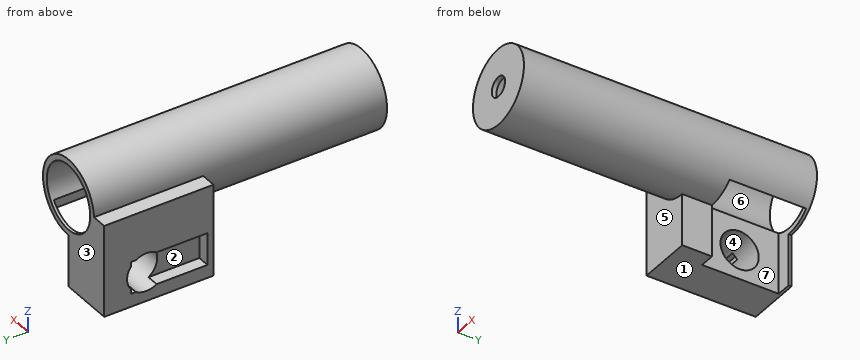
```python
from build123d import *

# Parameters (mm, degrees)
F0_R      = 25
F1_DEPTH  = 200
F4_W      = 35
F4_H      = 60
F5_DEPTH  = 80
F2_R      = 21.25
F6_DEPTH  = 197
F3_W      = 27
F3_H      = 50
F8_DEPTH  = 60
F9_DEPTH  = 8
F10_W     = 47.1464432776
F10_H     = 8.6505031213
F10_W_2   = 35
F12_DEPTH = 83.7927124713
F14_DEPTH = 50
F15_R     = 6.4891960767
F16_DEPTH = 25


with BuildPart() as f1:
    # F0 (on Front) → F1 (new body)
    with BuildSketch(Plane.XZ):
        Circle(F0_R)
    extrude(amount=F1_DEPTH)

    # F4 (on Front) → F5 (join)
    with BuildSketch(Plane.XZ):
        with Locations((-17.5, -28.7917124713)):
            Rectangle(F4_W, F4_H)
    extrude(amount=F5_DEPTH)

    # F2 (on face) → F6 (cut)
    with BuildSketch(Plane(origin=(0, 0, 0), x_dir=(-1, 0, 0), z_dir=(0, 1, 0))):
        Circle(F2_R)
    extrude(amount=-F6_DEPTH, mode=Mode.SUBTRACT)

    # F3 (on Top) → F8 (cut)
    with BuildSketch(Plane.XY):
        with Locations((3.8086780198, -35.5690324024)):
            Rectangle(F3_W, F3_H)
    extrude(amount=-F8_DEPTH, mode=Mode.SUBTRACT)

    # F7 (on face) → F9 (cut)
    with BuildSketch(Plane(origin=(-35, 0, 0), x_dir=(0, -1, 0), z_dir=(-1, 0, 0))):
        with BuildLine():
            ThreePointArc((41.3552170133, -29.25), (46.082189469, -33.5816991961), (47.8314612359, -39.75))
            ThreePointArc((47.8314612359, -39.75), (46.082189469, -45.9183008039), (41.3552170133, -50.25))
            Line((41.3552170133, -50.25), (76.0814612359, -50.25))
            Line((76.0814612359, -50.25), (76.0814612359, -29.25))
            Line((76.0814612359, -29.25), (41.3552170133, -29.25))
        make_face()
        with BuildLine():
            Line((26.0814612359, -50.25), (30.8077054584, -50.25))
            ThreePointArc((30.8077054584, -50.25), (28.1435615229, -48.4132700608), (26.0814612359, -45.9194813396))
            Line((26.0814612359, -45.9194813396), (26.0814612359, -50.25))
        make_face()
        with BuildLine():
            Line((36.0814612359, -29.25), (30.8077054584, -29.25))
            ThreePointArc((30.8077054584, -29.25), (28.1435615229, -31.0867299392), (26.0814612359, -33.5805186604))
            Line((26.0814612359, -33.5805186604), (26.0814612359, -45.9194813396))
            ThreePointArc((26.0814612359, -45.9194813396), (28.1435615229, -48.4132700608), (30.8077054584, -50.25))
            Line((30.8077054584, -50.25), (36.0814612359, -50.25))
            Line((36.0814612359, -50.25), (36.0814612359, -29.25))
        make_face()
        with BuildLine():
            ThreePointArc((26.0814612359, -33.5805186604), (28.1435615229, -31.0867299392), (30.8077054584, -29.25))
            Line((30.8077054584, -29.25), (26.0814612359, -29.25))
            Line((26.0814612359, -29.25), (26.0814612359, -33.5805186604))
        make_face()
    extrude(amount=-F9_DEPTH, mode=Mode.SUBTRACT)

    # F10 (on face) → F12 (cut, through all)
    with BuildSketch(Plane(origin=(0, 0, -58.7917124713), x_dir=(1, 0, 0), z_dir=(0, 0, -1))):
        with Locations((23.5732216388, 4.3252515607)):
            Rectangle(F10_W, F10_H)
        with Locations((-17.5, 4.3252515607)):
            Rectangle(F10_W_2, F10_H)
    extrude(amount=-F12_DEPTH, mode=Mode.SUBTRACT)

    # F13 (on face) → F14 (cut)
    with BuildSketch(Plane(origin=(-35, 0, 0), x_dir=(0, -1, 0), z_dir=(-1, 0, 0))):
        with BuildLine():
            ThreePointArc((23.5814612359, -39.75), (36.0814612359, -52.25), (48.5814612359, -39.75))
            ThreePointArc((48.5814612359, -39.75), (36.0814612359, -27.25), (23.5814612359, -39.75))
        make_face()
    extrude(amount=-F14_DEPTH, mode=Mode.SUBTRACT)

    # F15 (on face) → F16 (cut)
    with BuildSketch(Plane.XZ.offset(200)):
        Circle(F15_R)
    extrude(amount=-F16_DEPTH, mode=Mode.SUBTRACT)


solid = f1.part
```
CAD build for the part. Positions are in the model's coordinates, mm. Face numbers are marked on the shaded views. A direction names the side the tool comes from. Round coordinates to 2 decimals unless told otherwise and drop trailing zeros. Order: outer loops, then holes, each group sorted by start corner. A loop starts at its lowest first (then second) coordinate and runs counter-clockwise, first axis right, second up.
Q1. Which spindle directions (+Z, -Z, +X, -X, +Y, -Y) get a long thin tool onto all of the face, cutting with end or side? Do the marked faces 5, 6 and 7. Say none if no direction does.
Q2. Slice it at A-A (z = -39.75). Write the cut outline in (x, y).
Q3. Slice it at D-D (x = 14). Write the cut outline in (y, z).
Q4. Wall check: L1, parallel to Y at x = -0.5, z = -40.5; L2, parallel to Y at x = -21, z = -39; L3, parallel to Z at x = 0, y = -103. Give the ranges that are in metal, low to high.
Q5. Slice it at B-B (y = -71). Write the cut outline in (x, z), and give its area (3 significant figures).
Q6. Slice it at C-C (x = -4). Write the cut outline in (y, z).
Q7. Two-plate mould, pull along Z, no slides. Class the marked faces 1, 2, 3 and 4: pulls with the +Z half, pulls with the -Z half, needs draft (parallel to the pull), parting line crosses it, or undercut.
Q8. Drop flat-ended pins along their axis: pin 1 (10 mm diameter, centred on y = -40, z = 9.5, fed in from -X); pin 2 (5 mm diameter, centred on x = -30, y = -59, fed in from +Z); pin 3 (6.5 mm diameter, centred on y = -62.5, z = -40, fed in from -X); pin 4 (4 mm diameter, centred on x = -25, z = -8.5, fed in from -Y). Give the stop position or say it passes through.
Results below:
1. face 5: -Z, -X, -Y
1. face 6: +Y
1. face 7: -Z, +X
2. outline: (-35, -80) - (0, -80) - (0, -60.57) - (-9.69, -60.57) - (-9.69, -48.58) - (-27, -48.58) - (-27, -76.08) - (-35, -76.08) - close; (-35, -23.58) - (-9.69, -23.58) - (-9.69, -10.57) - (0, -10.57) - (0, -8.65) - (-35, -8.65) - close
3. outline: (-200, -20.71) - (-60.57, -20.71) - (-60.57, -15.99) - (-197, -15.99) - (-197, 15.99) - (-8.65, 15.99) - (-8.65, 20.71) - (-200, 20.71) - close; (-10.57, -20.71) - (-8.65, -20.71) - (-8.65, -15.99) - (-10.57, -15.99) - close
4. L1: y = -80 to -60.57, -10.57 to -8.65
4. L2: y = -80 to -48.56, -23.6 to -8.65
4. L3: z = -25 to -21.25, 21.25 to 25
5. outline: (-35, -58.79) - (0, -58.79) - (0, -25) arc R25 ccw (long way) to (-24.97, 1.21) - (-35, 1.21) - (-35, -29.25) - (-27, -29.25) - (-27, -50.25) - (-35, -50.25) - close; hole circle Ø42.5 at (0, 0)
5. area: 1,960 mm2
6. outline: (-200, -24.68) - (-80, -24.68) - (-80, -58.79) - (-60.57, -58.79) - (-60.57, -20.87) - (-197, -20.87) - (-197, -5.11) - (-200, -5.11) - close; (-200, 5.11) - (-197, 5.11) - (-197, 20.87) - (-8.65, 20.87) - (-8.65, 24.68) - (-200, 24.68) - close; (-10.57, -58.79) - (-8.65, -58.79) - (-8.65, -20.87) - (-10.57, -20.87) - close
7. face 1: pulls with the -Z half
7. face 2: undercut
7. face 3: needs draft
7. face 4: undercut
8. pin 1: stops at x = -24.59
8. pin 2: stops at z = 1.21
8. pin 3: stops at x = -27
8. pin 4: stops at y = -200
